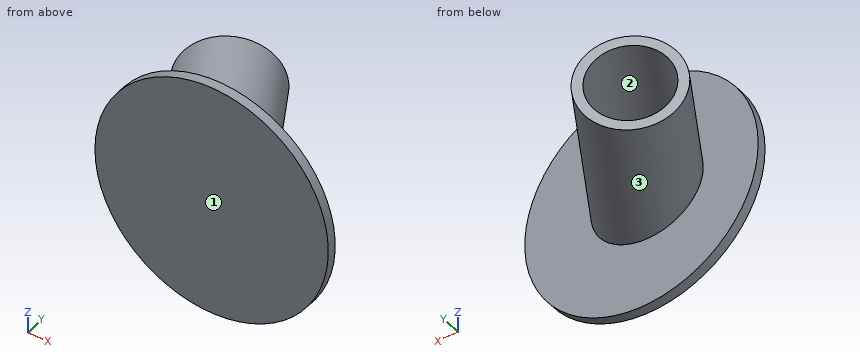
from build123d import *

# Parameters (mm, degrees)
F2_R          = 38.1
F3_DEPTH      = 3.175
F6_R          = 15.875
F6_R_2        = 12.7
F7_DEPTH      = 50.8
F7_DEPTH_BACK = 6.35
F9_DEPTH      = 25.4
F9_DEPTH_BACK = 25.4


with BuildPart() as f3:
    # F2 (on line) → F3 (new body)
    with BuildSketch(Plane(origin=(0, 0, 0), x_dir=(-1, 0, 0), z_dir=(0, 1, 0))):
        Circle(F2_R)
    extrude(amount=F3_DEPTH)

    # F6 (on line) → F7 (join, two sides)
    with BuildSketch(Plane(origin=(0, 0, 0), x_dir=(-0.8660254038, -0.5, 0), z_dir=(-0.5, 0.8660254038, 0))) as f7_sk:
        Circle(F6_R)
        Circle(F6_R_2, mode=Mode.SUBTRACT)
    extrude(amount=F7_DEPTH)
    extrude(f7_sk.sketch, amount=-F7_DEPTH_BACK)

    # F8 (on Right) → F9 (cut, two sides)
    with BuildSketch(Plane.YZ) as f9_sk:
        Polygon((0, -20.3028712422), (0, 23.2852003007), (-20.0170747743, 19.199454845), (-8.2928827169, -22.6273914554), align=None)
    extrude(amount=-F9_DEPTH, mode=Mode.SUBTRACT)
    extrude(f9_sk.sketch, amount=F9_DEPTH_BACK, mode=Mode.SUBTRACT)


solid = f3.part
Here's how the part is built. I have some questions about the finished solid (model axes, mm). Face numbers are marked on the shaded views. Round coordinates to 2 decimals unless told otherwise and drop trailing zeros. Loops run counter-clockwise (first coordinate to the right, second up) from the corner with the lowest first, then second, coordinate; pieces in that order, holes last. Notation, with made-up numbers: (11.5, 89) - (30.5, 89) arc R19 ccw to (30.5, 110) - close; hole circle Ø7 at (50, 34.5). An arc over 180 degrees is marked (long way). One line per question, with ' | ' between items. Start each with the question number.
Q1. I want a section at A-A (z = -5.5). Write out the boundary of the cut face in (x, y) (3 decimals).
Q2. Please list where these lines run through material, in increasing order: line 1 (Y direction, x = -23.5, z = 5) (3 decimals); line 2 (Y direction, x = 31, z = -1) (3 decimals); line 3 (X direction, y = 11, z = -2.5). Write a range as [from, to].
Q3. We'd pull the mould along Y, two halves only. Please class the marked faces 1, 2 and 3: +Y half, -Y half, draft (parallel to the pull), parting line (faces both ways), or undercut.
Q4. I want a section at C-C (z = 10). Write out the boundary of the cut face in (x, y) (3 decimals).
Q5. I want a section at B-B (x = 32). Write out the boundary of the cut face in (y, z) (3 decimals).
Q6. Will these pins go through, and if not, where does the flat tip stop? pin 1 (10 mm diameter, centred on x = -29.5, y = 21.5, fed in from -Z); pin 2 (8 mm diameter, centred on x = -3.5, z = -24.5, fed in from +Y) (3 decimals); pin 3 (10 mm diameter, centred on x = -31, y = 9, fed in from +Z); pin 4 (3 mm diameter, centred on x = -19, y = 22.5, fed in from +Z).
Q7. I want a section at D-D (z = 22). Write out the boundary of the cut face in (x, y) (3 decimals), then the cut area to 3 significant figures.
Response values:
1) outline: (-38.297, 36.548) - (-19.029, 3.175) - (-37.701, 3.175) - (-37.701, 0) - (37.701, 0) - (37.701, 3.175) - (15.362, 3.175) - (-12.503, 51.44) - (-15.486, 49.718) - (11.385, 3.175) - (-15.051, 3.175) - (-35.314, 38.27) - close
2) line 1: y = [0, 3.175], [10.569, 17.355] | line 2: y = [0, 3.175] | line 3: x = [-24.45, -20.73], [8.03, 11.75]
3) face 1: -Y half | face 2: undercut | face 3: undercut
4) outline: (-36.764, 0) - (36.764, 0) - (36.764, 3.175) - (12.404, 3.175) - (-14.722, 50.159) - (-18.62, 47.908) - (7.207, 3.175) - (-10.873, 3.175) - (-32.18, 40.08) - (-36.078, 37.829) - (-16.07, 3.175) - (-36.764, 3.175) - close
5) outline: (0, -20.679) - (3.175, -20.679) - (3.175, 20.679) - (0, 20.679) - close
6) pin 1: stops at z = -12.49 | pin 2: stops at y = 3.175 | pin 3: passes through | pin 4: stops at z = 15.44
7) outline: (-31.106, 0) - (31.106, 0) - (31.106, 3.175) - (-31.106, 3.175) - close | area: 198 mm²
